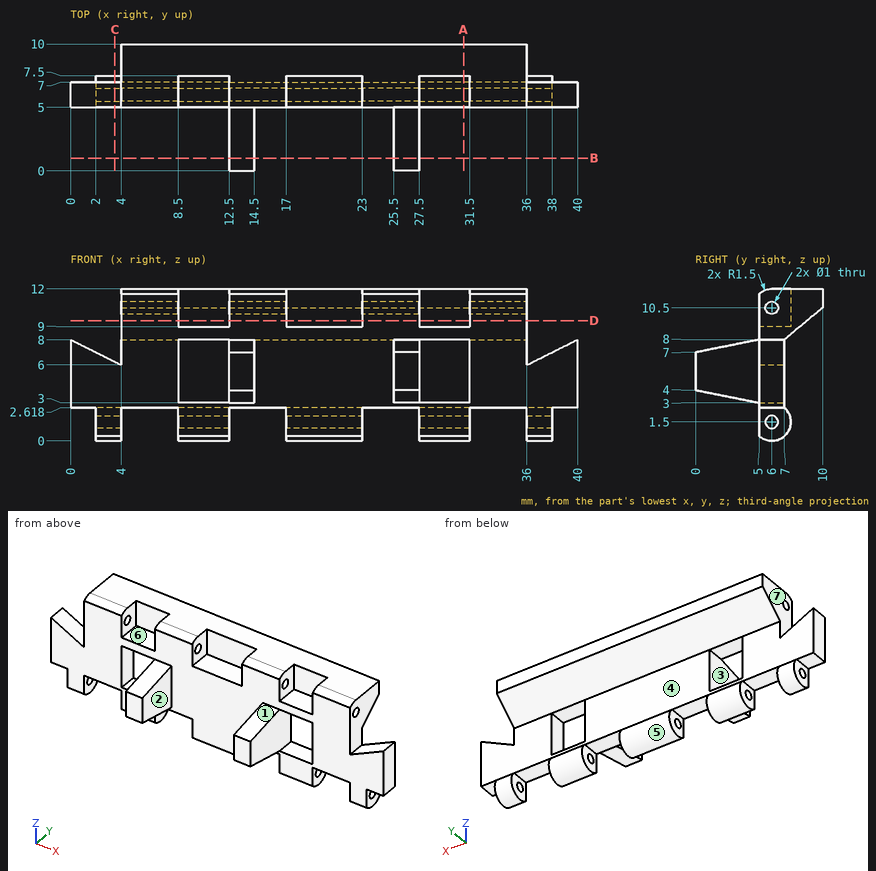
Job drawing, mm, ordinate dimensions from the low corner. One solid piece. A direction names the side the tool comes from. Give positions to 0.01 mm unless a question says otherwise; leave off trailing zeros. Order: outer loops, then holes, each group sorted by start corner. A loop starts at its lowest first (then second) coordinate and runs counter-clockwise, first axis right, second up. Notation, with made-up numbers: (-10, 20) -> (7, 20) arc R21 ccw to (7, 34) -> close; hole circle Ø11 at (63, 59). An arc over 180 degrees is marked (long way). Return JSON: item names as keys, results as strings.
Q1. Saw through at A-A (x = 31). Write the cut outline in (y, z).
Working result:
{"outline": "(5, 0.38) arc R1.5 ccw to (7, 2.62) -> (7, 3) -> (5, 3) -> close; (5, 8) -> (7, 8) -> (10, 10.5) -> (10, 12) -> (7.5, 12) -> (7.5, 9) -> (5, 9) -> close; hole circle Ø1 at (6, 1.5)"}
Q2. Drill centre lines: line 1 (X direction, y = 4.5, z = 5.5); line 2 (Y direction, x = 21.85, z = 1.5); line 3 (X direction, y = 8.25, z = 10.25). Where is each one in solid material? Low to high.
Working result:
{"line 1": "12.5 to 14.5, 25.5 to 27.5", "line 2": "5 to 5.5, 6.5 to 7.5", "line 3": "4 to 36"}
Q3. Which spindle directions (+Z, -Z, +X, -X, +Y, -Y) get a long thin tool onto all of the face, cutting with end or side? Do the marked faces 3, 4, 5, 6 and 7. Say none if no direction does.
Working result:
{"face 3": "+Y, -Y", "face 4": "+X, -X, +Y", "face 5": "+X, -X", "face 6": "+Z, -Y", "face 7": "+Z, +Y, -Y"}
Q4. Saw through at C-C (x = 3.5). Write the cut outline in (y, z), then the cut area to 4 significant figures.
Working result:
{"outline": "(5, 0.38) arc R1.5 ccw to (7, 2.62) -> (7, 6.25) -> (5, 6.25) -> close; hole circle Ø1 at (6, 1.5)", "area": "12.25 mm²"}
Q5. Flat gauge pins, fed straight in: pin 1 (4 mm diameter, centred on y = 2, z = 3.5, fed in from +X); pin 2 (3 mm diameter, centred on y = 6, z = 1, fed in from +X); pin 3 (1.5 mm diameter, centred on x = 32.5, z = 9.5, fed in from -Y). Where does each tip first touch, or does it go through?
Working result:
{"pin 1": "x = 27.5", "pin 2": "x = 38", "pin 3": "y = 5"}
Q6. Saw through at B-B (y = 1). Write the cut outline in (x, z), then the cut area to 3 significant figures.
Working result:
{"outline": "(12.5, 3.8) -> (14.5, 3.8) -> (14.5, 7.2) -> (12.5, 7.2) -> close; (25.5, 3.8) -> (27.5, 3.8) -> (27.5, 7.2) -> (25.5, 7.2) -> close", "area": "13.6 mm²"}
Q7. Saw through at D-D (z = 9.5). Write the cut outline in (x, y), then the cut area to 3 significant figures.
Working result:
{"outline": "(4, 5) -> (8.5, 5) -> (8.5, 7.5) -> (12.5, 7.5) -> (12.5, 5) -> (17, 5) -> (17, 7.5) -> (23, 7.5) -> (23, 5) -> (27.5, 5) -> (27.5, 7.5) -> (31.5, 7.5) -> (31.5, 5) -> (36, 5) -> (36, 8.8) -> (4, 8.8) -> close", "area": "86.6 mm²"}
Q8. Mould opens along X. For the marked faces 1 and 2 say: pulls with the +X half, pulls with the -X half, needs draft (parallel to the pull), parting line crosses it, or undercut.
Working result:
{"face 1": "needs draft", "face 2": "undercut"}
